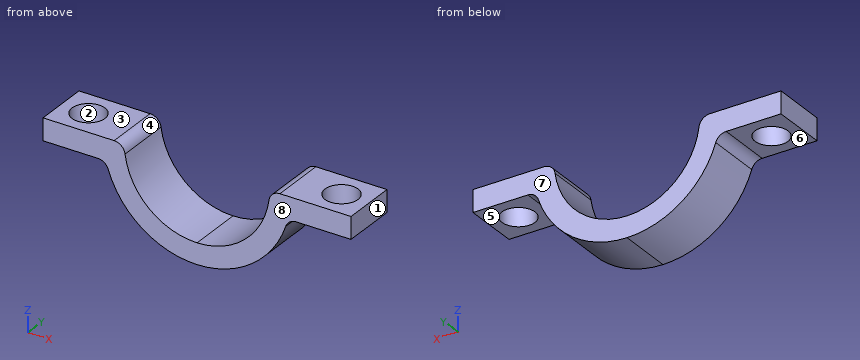
from build123d import *

# Parameters (mm, degrees)
BOSS_EXTRUDE1_DEPTH = 5
SKETCH2_R           = 1.5
CUT_EXTRUDE1_DEPTH  = 17.22498074
FILLET1_R           = 1


with BuildPart() as part:
    # Sketch1 → Boss-Extrude1 (new body)
    with BuildSketch(Plane(origin=(0, 0, 0), x_dir=(1, 0, 0), z_dir=(0, 1, 0))):
        with BuildLine():
            Line((-14, 0), (-8.5, 0))
            Line((-8.5, 0), (-6.6, 0))
            ThreePointArc((-6.6, 0), (-4.666904756, 4.666904756), (0, 6.6))
            Line((0, 6.6), (0, 8.5))
            ThreePointArc((0, 8.5), (-5.25594901, 6.680194608), (-8.261355821, 2))
            Line((-8.261355821, 2), (-14, 2))
            Line((-14, 2), (-14, 0))
        make_face()
        with BuildLine():
            Line((0, 8.5), (0, 6.6))
            ThreePointArc((0, 6.6), (4.666904756, 4.666904756), (6.6, 0))
            Line((6.6, 0), (8.5, 0))
            Line((8.5, 0), (14, 0))
            Line((14, 0), (14, 2))
            Line((14, 2), (8.261355821, 2))
            ThreePointArc((8.261355821, 2), (5.25594901, 6.680194608), (0, 8.5))
        make_face()
    extrude(amount=BOSS_EXTRUDE1_DEPTH)

    # Sketch2 → Cut-Extrude1 (cut, through all)
    with BuildSketch(Plane(origin=(0, 0, -2), x_dir=(-1, 0, 0), z_dir=(0, 0, -1))):
        with Locations((-11.5, 2.5)):
            Circle(SKETCH2_R)
        with Locations(Location((11.5, 2.5, 0), (0, 0, 180))):
            Circle(SKETCH2_R)
    extrude(amount=-CUT_EXTRUDE1_DEPTH, mode=Mode.SUBTRACT)

    # Fillet1
    fillet1_edges = [part.edges().sort_by_distance(p)[0] for p in [
        (-6.6, 2.5, 0),
        (-8.261355821, 2.5, -2),
        (8.261355821, 2.5, -2),
        (6.6, 2.5, 0),
    ]]
    fillet(fillet1_edges, radius=FILLET1_R)


solid = part.part
The listing builds one solid part. Answer for the finished solid, in the listing's coordinates (mm). Face numbers are marked on the shaded views. A direction names the side the tool comes from. Give positions to 0.01 mm unless a question says otherwise; leave off trailing zeros. Loops run counter-clockwise (first coordinate to the right, second up) from the corner with the lowest first, then second, coordinate; pieces in that order, holes last. Notation, with made-up numbers: (-7, 18.25) - (24, 18.25) arc R18 cw to (24, 38.25) - close; hole circle Ø8 at (84, 68.5). An arc over 180 degrees is marked (long way). Write each question's results on one line, items separated by ' | '.
1. Flat-ended cylindrical pins translate along their axes: P1, Ø3, axis at y = 3, z = -6.5, coming from the +X side; P2, Ø2.5, axis at x = -11.5, y = 2, coming from the -Z side. Find the tip coordinate at first contact, or state that the pin passes through.
Resolved:
P1: stops at x = 6.87 | P2: stops at z = -2
2. For a pull along X with two mould halves and no side action, classify the marked faces 1, 2 and 3 as +X half, -X half, draft (parallel to the pull), parting line (faces both ways), or undercut.
Resolved:
face 1: +X half | face 2: undercut | face 3: draft
3. Find section D-D, the plane z = -1.5. Write down the section's boundary in (x, y).
Resolved:
outline: (-14, 0) - (-6.43, 0) - (-6.43, 5) - (-14, 5) - close; (6.43, 0) - (14, 0) - (14, 5) - (6.43, 5) - close; hole circle Ø3 at (-11.5, 2.5); hole circle Ø3 at (11.5, 2.5)
4. Find section B-B, the plane y = 2.5. Write down the section's boundary in (x, z).
Resolved:
outline: (-14, -2) - (-13, -2) - (-13, 0) - (-14, 0) - close; (-10, -2) - (-9.01, -2) arc R1 cw to (-8.07, -2.68) arc R8.5 ccw to (8.07, -2.68) arc R1 cw to (9.01, -2) - (10, -2) - (10, 0) - (7.53, 0) arc R1 ccw to (6.54, -0.87) arc R6.6 cw to (-6.54, -0.87) arc R1 ccw to (-7.53, 0) - (-10, 0) - close; (13, -2) - (14, -2) - (14, 0) - (13, 0) - close
5. Which of the six approach directions +Z, -Z, +X, -X, +Y, -Y give full straight-line access (tool end or side, diameter ignored) to the marked faces 4, 5, 6, 7 and 8?
Resolved:
face 4: +Z, +Y, -Y | face 5: -Z, +X, +Y, -Y | face 6: -Z, -X, +Y, -Y | face 7: +Z, -Z, +X, -X, +Y | face 8: +Z, -Z, +X, -X, -Y
6. Consider probe 1 along Y at (x, z) = (-11.5, -1); probe 2 along X at (y, z) = (1.35, -0.5); probe 3 along X at (y, z) = (0.4, -4.5). Determine where each line is inside the solid, lowest interval first. Write a range as from..to.
Resolved:
probe 1: y = 0..1, 4..5 | probe 2: x = -14..-12.46, -10.54..-6.67, 6.67..10.54, 12.46..14 | probe 3: x = -7.21..-4.83, 4.83..7.21
7. Find section C-C, the plane z = -3. Write down the section's boundary in (x, y), then the cut area to 3 significant figures.
Resolved:
outline: (-7.95, 0) - (-5.88, 0) - (-5.88, 5) - (-7.95, 5) - close; (5.88, 0) - (7.95, 0) - (7.95, 5) - (5.88, 5) - close | area: 20.7 mm^2
8. Find section A-A, the plane x = 11.5. Write down the section's boundary in (y, z), then the cut area to 3 significant figures.
Resolved:
outline: (0, -2) - (1, -2) - (1, 0) - (0, 0) - close; (4, -2) - (5, -2) - (5, 0) - (4, 0) - close | area: 4.00 mm^2
